For this review, take the finished solid that the model builds, in its own axes (mm). Face numbers are marked on the shaded views. A direction names the side the tool comes from. Coordinates: 2 decimals unless noted, no trailing zeros. Order: outer loops, then holes, each group sorted by start corner. A loop starts at its lowest first (then second) coordinate and runs counter-clockwise, first axis right, second up.
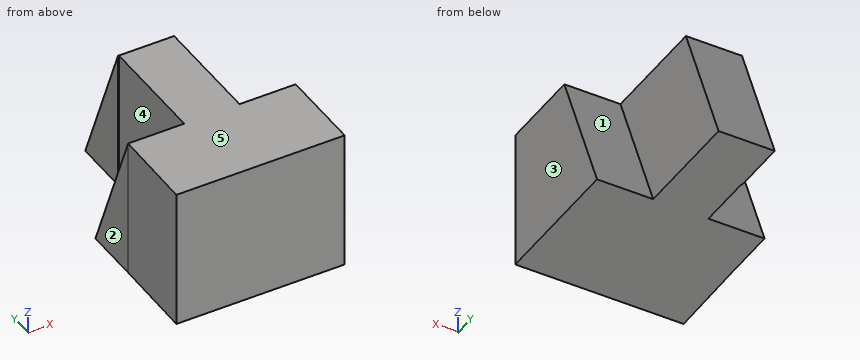
from build123d import *

# Parameters (mm, degrees)
F1_DEPTH = 31.75
F3_DEPTH = 12.7
F5_DEPTH = 12.7
F7_DEPTH = 12.7


with BuildPart() as f1:
    # F0 (on Top) → F1 (new body)
    with BuildSketch(Plane.XY):
        Polygon((-53.184141, -37.298974), (-53.380532, -56.348974), (-15.280532, -56.348974), (-15.280532, -37.298974), (-27.980532, -37.298974), (-27.980532, -11.898974), (-40.484141, -11.898974), (-40.484141, -37.298974), align=None)
    extrude(amount=F1_DEPTH)

    # F2 (on face) → F3 (join)
    with BuildSketch(Plane.YZ.offset(-27.980532)):
        Polygon((-24.598974, 0), (-37.298974, 31.75), (-37.298974, 0), align=None)
    extrude(amount=F3_DEPTH)

    # F4 (on face) → F5 (join)
    with BuildSketch(Plane(origin=(-40.484141, 0, 0), x_dir=(0, -1, 0), z_dir=(-1, 0, 0))):
        Polygon((37.298974, 0), (37.298974, 31.75), (24.598974, 0), align=None)
    extrude(amount=F5_DEPTH)

    # F6 (on face) → F7 (join)
    with BuildSketch(Plane.YZ.offset(-27.980532)):
        Polygon((0.801026, 0), (-11.898974, 31.75), (-11.898974, 0), align=None)
    extrude(amount=-F7_DEPTH)


solid = f1.part
1. Take a section at A-A, the plane z = 25.5. Give the boundary of the cut face in (x, y), plus the area to 3 significant figures.
Answer below:
outline: (-53.38, -56.35) - (-15.28, -56.35) - (-15.28, -34.8) - (-27.98, -34.8) - (-27.98, -9.4) - (-40.68, -9.4) - (-40.68, -11.9) - (-40.48, -11.9) - (-40.48, -34.8) - (-53.18, -34.8) - (-53.18, -37.3) - close
area: 1,140 mm2
2. Take a section at B-B, the plane x = -42.5. Give the boundary of the cut face in (y, z), plus the area to 3 significant figures.
Answer below:
outline: (-56.35, 0) - (-24.6, 0) - (-37.3, 31.75) - (-56.35, 31.75) - close
area: 806 mm2
3. Clearance check with flat-ended pins moving along their axes: pin 1 Ø2 at (x, z) = (-26.5, 12.5) entering from +Y; pin 2 Ø14 at (y, z) = (-8, 13) entering from -X; pin 3 Ø10 at (y, z) = (-29.5, 19.5) entering from -X. State where each tip first meets the part, or that it passes through.
Answer below:
pin 1: stops at y = -29.2
pin 2: stops at x = -40.68
pin 3: stops at x = -53.18
4. Take a section at C-C, the plane y = -14. Give the boundary of the cut face in (x, z).
Answer below:
outline: (-40.48, 0) - (-27.98, 0) - (-27.98, 31.75) - (-40.48, 31.75) - close
5. Take a section at D-D, the plane z = 9.5. Give the boundary of the cut face in (x, y), plus the area to 3 significant figures.
Answer below:
outline: (-53.38, -56.35) - (-15.28, -56.35) - (-15.28, -28.4) - (-27.98, -28.4) - (-27.98, -3) - (-40.68, -3) - (-40.68, -11.9) - (-40.48, -11.9) - (-40.48, -28.4) - (-53.18, -28.4) - (-53.18, -37.3) - close
area: 1,380 mm2
6. To check wall thickness, follow L1, parallel to X at y = -18.5, z = 27.5; L2, parallel to Y at x = -41, z = 26; L3, parallel to Y at x = -34.5, z = 3. State the ranges of each line that lie inside material, in increasing order.
Answer below:
L1: x = -40.48 to -27.98
L2: y = -56.35 to -35
L3: y = -56.35 to -0.4
7. Machinability: for the marked faces 1, 2, 3, 4 and 5, which of the approach directions +Z, -Z, +X, -X, +Y, -Y give a long, thin tool a straight path to every point of the face, cutting with its end or side? Answer none if there is none.
Answer below:
face 1: +Z, +X, +Y
face 2: +Z, -Z, -X, +Y
face 3: +Z, -Z, +X, +Y, -Y
face 4: +Z, -X
face 5: +Z, +X, -X, +Y, -Y
